Geometry check sheet. Reference: drawing and pictorial views, mm from the part's lowest x, y, z. A direction names the side the tool comes from. Coordinates: 2 decimals unless noted, no trailing zeros. Write each loop counter-clockwise with the first axis right and the second up, starting at its lowest first coordinate (ties: lowest second). Pieces come first, ordered by that corner, then holes. Notation, with made-up numbers: (85, -12) -> (89, -12) arc R10 cw to (89, 6) -> close; hole circle Ø9 at (22.5, -27). An arc over 180 degrees is marked (long way). Use a Markdown table: item, result. Add a question column.
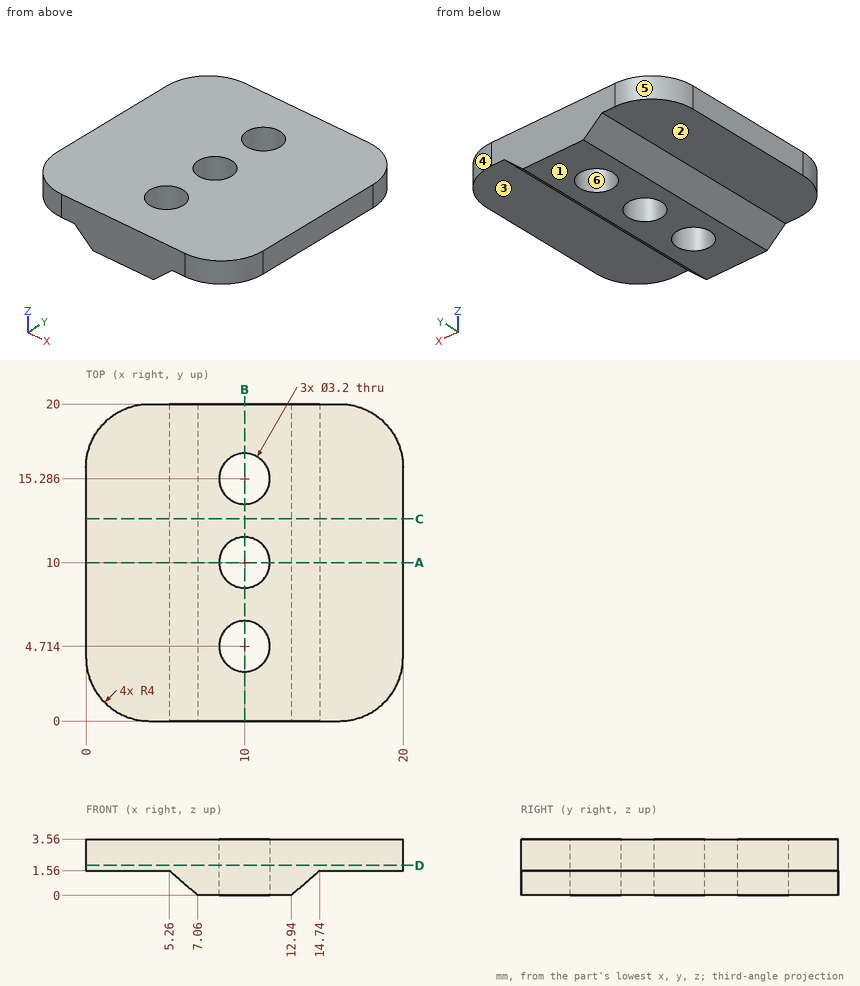
1) Cross-section at A-A on y = 10. Record the boundary of the cut face in (x, z), then the cut area to 3 significant figures.
2) Release check for a two-part mould opening along X. For the marked faces 4, 5 and 6 record: released by +X, released by -X, zero draft, split by the parting line, or undercut.
3) Thickness scan on L1, parallel to Y at x = 10, z = 0.85; L2, parallel to Z at x = 2, y = 19; L3, parallel to X at y = 10.25, z = 1.25. Record the ranges inside material, lowest first.
4) Set-up check for the marked faces 1, 2 and 3: record each of +Z, -Z, +X, -X, +Y, -Y from which the full face is reachable in a straight line by a thin tool's end or side.
5) Cross-section at C-C on y = 12.75. Record the boundary of the cut face in (x, z).
6) Gauge pin test, flat ends, axial feed: pin 1 (1 mm diameter, centred on y = 13.5, z = 1.5, fed in from -X); pin 2 (4 mm diameter, centred on x = 16, y = 10.5, fed in from -Z); pin 3 (6 mm diameter, centred on x = 2.5, y = 14.5, fed in from -Z); pin 4 (1.5 mm diameter, centred on x = 17.5, y = 2, fed in from -Z). Record the tip position at first contact, or that the pin passes through.
7) Cross-section at B-B on x = 10. Record the boundary of the cut face in (y, z), then the cut area to 3 significant figures.
8) Cross-section at D-D on z = 1.9. Record the boundary of the cut face in (x, y).
Returned:
| question | item | result |
|---|---|---|
| 1 | outline | (0, 1.56) -> (5.26, 1.56) -> (7.06, 0) -> (8.4, 0) -> (8.4, 3.56) -> (0, 3.56) -> close; (11.6, 0) -> (12.94, 0) -> (14.74, 1.56) -> (20, 1.56) -> (20, 3.56) -> (11.6, 3.56) -> close |
| 1 | area | 40.6 mm² |
| 2 | face 4 | released by +X |
| 2 | face 5 | released by -X |
| 2 | face 6 | undercut |
| 3 | L1 | y = 0 to 3.11, 6.31 to 8.4, 11.6 to 13.69, 16.89 to 20 |
| 3 | L2 | z = 1.56 to 3.56 |
| 3 | L3 | x = 5.62 to 8.42, 11.58 to 14.38 |
| 4 | face 1 | -Z, +X, -X, +Y, -Y |
| 4 | face 2 | -Z, -X, +Y, -Y |
| 4 | face 3 | -Z, +X, +Y, -Y |
| 5 | outline | (0, 1.56) -> (5.26, 1.56) -> (7.06, 0) -> (12.94, 0) -> (14.74, 1.56) -> (20, 1.56) -> (20, 3.56) -> (0, 3.56) -> close |
| 6 | pin 1 | stops at x = 0 |
| 6 | pin 2 | stops at z = 0.92 |
| 6 | pin 3 | stops at z = 1.35 |
| 6 | pin 4 | stops at z = 1.56 |
| 7 | outline | (0, 0) -> (3.11, 0) -> (3.11, 3.56) -> (0, 3.56) -> close; (6.31, 0) -> (8.4, 0) -> (8.4, 3.56) -> (6.31, 3.56) -> close; (11.6, 0) -> (13.69, 0) -> (13.69, 3.56) -> (11.6, 3.56) -> close; (16.89, 0) -> (20, 0) -> (20, 3.56) -> (16.89, 3.56) -> close |
| 7 | area | 37.0 mm² |
| 8 | outline | (0, 4) arc R4 ccw to (4, 0) -> (16, 0) arc R4 ccw to (20, 4) -> (20, 16) arc R4 ccw to (16, 20) -> (4, 20) arc R4 ccw to (0, 16) -> close; hole circle Ø3.2 at (10, 4.71); hole circle Ø3.2 at (10, 10); hole circle Ø3.2 at (10, 15.29) |
